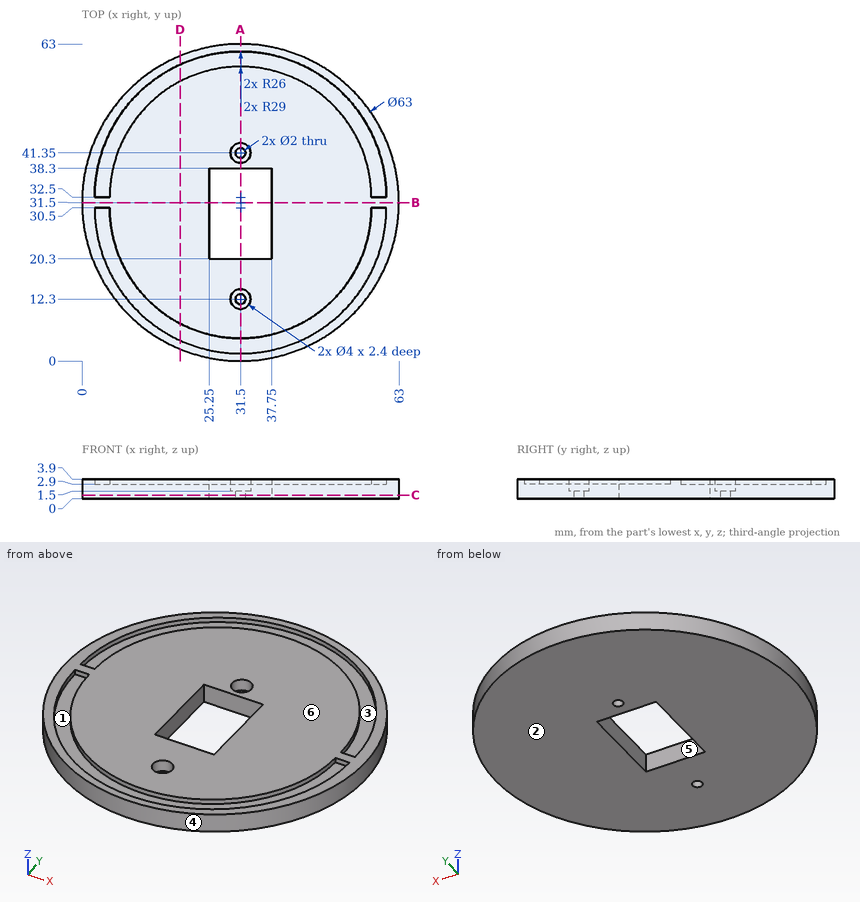
Answer from the drawing. Dimensions are ordinates in mm from the lowest x, y and z of the part. A direction names the side the tool comes from. Give positions to 0.01 mm unless a question says otherwise; leave off trailing zeros. Loops run counter-clockwise (first coordinate to the right, second up) from the corner with the lowest first, then second, coordinate; pieces in that order, holes last. Notation, with made-up numbers: (30, 88.25) -> (72, 88.25) arc R19 ccw to (72, 108.25) -> close; hole circle Ø8 at (75.5, 43). An arc over 180 degrees is marked (long way). One line per question, with ' | ' between items. Start each with the question number.
1) Section B-B, the plane y = 31.5 is taken. Determine the outline of the cut face in (x, z), then the cut area to 3 significant figures.
2) Section C-C, the plane z = 0.7 is taken. Determine the outline of the cut face in (x, y).
3) Each of these flat-tipped pins is pushed along its axis until it touches: pin 1 (1.1 mm diameter, centred on x = 4.5, z = 3, fed in from -Y); pin 2 (2 mm diameter, centred on x = 33, z = 1.5, fed in from +Y); pin 3 (1.2 mm diameter, centred on x = 32, y = 13, fed in from +Z). Where does it stop, or does it pass through?
4) For the marked faces 5 and 6, determine the directions among +Z, -Z, +X, -X, +Y, -Y from which every point of the face is accessible in a straight line to the end or side of a thin tool.
5) Section A-A, the plane x = 31.5 is taken. State how many separate pieces and enclosed holes the cut face has, then the cut area to 3 significant figures.
6) Section D-D, the plane x = 19.5 is taken. Determine the outline of the cut face in (y, z).
7) Straight lines are drawn through the part: L1, parallel to Y at x = 31.5, z = 2.1; L2, parallel to Y at x = 31.5, z = 1.15. For each, find the intervals that lie inside material, in ascending order.
8) Determine the mould class of the marked faces 1, 2, 3 and 4 for opening direction X: +X half, -X half, draft (parallel to the pull), parting line (faces both ways), or undercut.
Resolved:
1) outline: (0, 0) -> (25.25, 0) -> (25.25, 3.9) -> (0, 3.9) -> close; (37.75, 0) -> (63, 0) -> (63, 3.9) -> (37.75, 3.9) -> close | area: 197 mm2
2) outline: circle Ø63 at (31.5, 31.5); hole (25.25, 20.3) -> (37.75, 20.3) -> (37.75, 38.3) -> (25.25, 38.3) -> close; hole circle Ø2 at (31.5, 12.3); hole circle Ø2 at (31.5, 41.35)
3) pin 1: y = 14.39 | pin 2: y = 63 | pin 3: z = 1.5
4) face 5: +Z, -Z | face 6: +Z, +X, -X, +Y, -Y
5) separate pieces: 4 | enclosed holes: 0 | area: 144 mm2
6) outline: (2.38, 0) -> (60.62, 0) -> (60.62, 3.9) -> (58.9, 3.9) -> (58.9, 2.9) -> (55.57, 2.9) -> (55.57, 3.9) -> (7.43, 3.9) -> (7.43, 2.9) -> (4.1, 2.9) -> (4.1, 3.9) -> (2.38, 3.9) -> close
7) L1: 0 to 10.3, 14.3 to 20.3, 38.3 to 39.35, 43.35 to 63 | L2: 0 to 11.3, 13.3 to 20.3, 38.3 to 40.35, 42.35 to 63
8) face 1: undercut | face 2: draft | face 3: undercut | face 4: parting line
